The figure shows three views and two pictorial views of one solid part (mm, origin at its lowest corner). Answer the questions. Give positions to 0.01 mm unless a question says otherwise; leave off trailing zeros. Loops run counter-clockwise (first coordinate to the right, second up) from the corner with the lowest first, then second, coordinate; pieces in that order, holes last. Notation, with made-up numbers: M 30,19 L 55,19 A18 ccw 55,38 Z; hole C -23,-21 d6. An arc over 180 degrees is marked long. Write item = value, one per line. Start each with the question number.
1. Section B-B on x = 62.5 is taken. Determine the outline of the cut face in (y, z) (1 decimal).
2. Consider L1, parallel to X at y = 4, z = 78.5 (1 decimal); L2, parallel to X at y = 1.25, z = 56.5 (1 decimal); L3, parallel to Z at x = 62.5, y = 0.8 (1 decimal). Determine where each line is inside the solid, lowest interval first. Write a range as [from, to].
3. Section A-A on z = 44.25 is taken. Determine the outline of the cut face in (x, y).
4. Section C-C on z = 61 is taken. Determine the outline of the cut face in (x, y).
5. The mould has two halves that part along X. Classify the marked faces 1, 2, 3 and 4: released by +X, released by -X, zero draft, split by the parting line, or undercut.
6. Flat-ended cylindrical pins translate along their axes: pin 1 Ø5 at (x, z) = (16, 67) entering from +Y; pin 2 Ø1.8 at (x, z) = (63.5, 76.5) entering from +Y; pin 3 Ø9.5 at (x, z) = (37.91, 80.2) entering from -Y; pin 4 Ø4 at (x, y) = (25, 2.5) entering from -Z. Find the tip coordinate at first contact, or state that the pin passes through.
7. Section D-D on y = 3.75 is taken. Give the number of separate pieces and of enclosed holes in the cut face, plus the area to 3 significant figures.
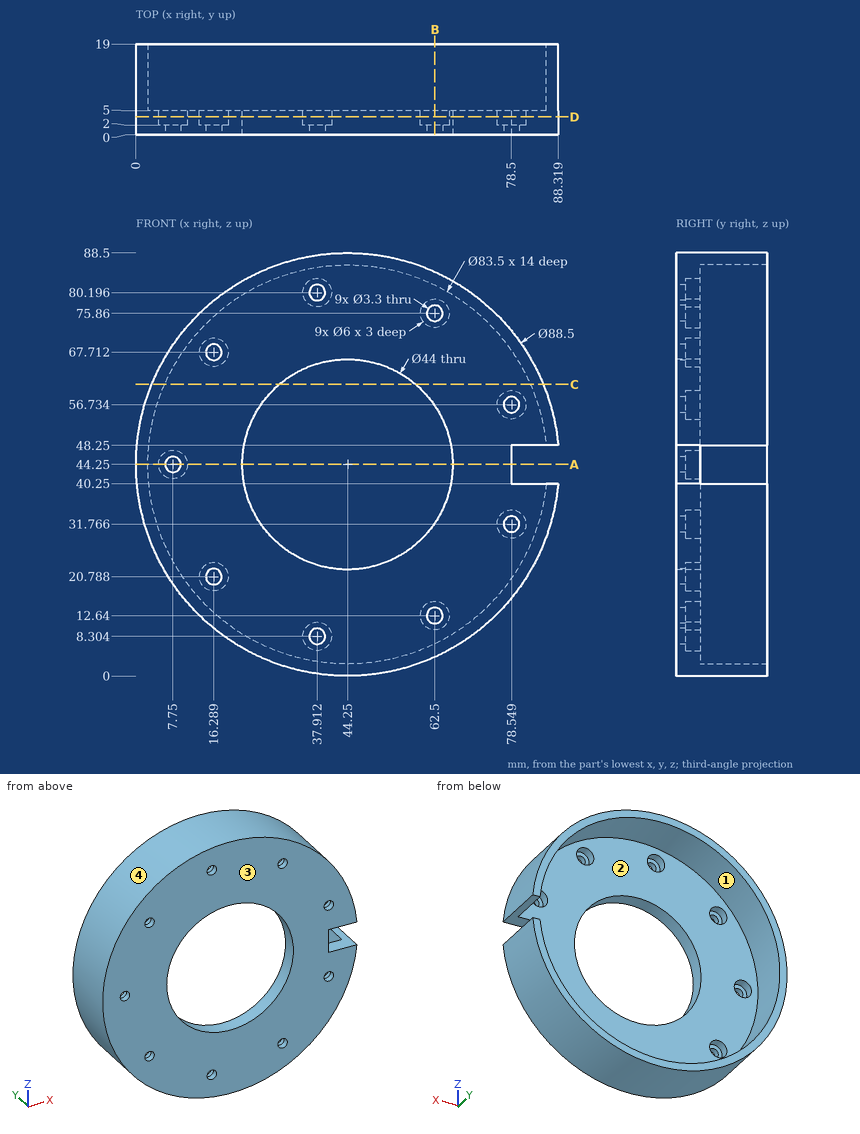
Verdict:
q1.outline = M 0,3.9 L 19,3.9 L 19,6.7 L 5,6.7 L 5,9.6 L 2,9.6 L 2,11 L 0,11 Z; M 0,14.3 L 2,14.3 L 2,15.6 L 5,15.6 L 5,32 L 0,32 Z; M 0,56.5 L 5,56.5 L 5,72.9 L 2,72.9 L 2,74.2 L 0,74.2 Z; M 0,77.5 L 2,77.5 L 2,78.9 L 5,78.9 L 5,81.8 L 19,81.8 L 19,84.6 L 0,84.6 Z
q2.L1 = [16.2, 35.4], [40.4, 61.1], [63.9, 72.3]
q2.L2 = [1.7, 26], [62.5, 76.9], [80.2, 86.8]
q2.L3 = [3.9, 11], [14.3, 32], [56.5, 74.2], [77.5, 84.6]
q3.outline = M 0,0 L 6.1,0 L 6.1,2 L 4.75,2 L 4.75,5 L 2.5,5 L 2.5,19 L 0,19 Z; M 9.4,0 L 22.25,0 L 22.25,5 L 10.75,5 L 10.75,2 L 9.4,2 Z; M 66.25,0 L 78.5,0 L 78.5,5 L 66.25,5 Z
q4.outline = M 3.29,0 L 29.99,0 L 29.99,5 L 6.01,5 L 6.01,19 L 3.29,19 Z; M 58.51,0 L 85.21,0 L 85.21,19 L 82.49,19 L 82.49,5 L 58.51,5 Z
q5.face_1 = undercut
q5.face_2 = undercut
q5.face_3 = zero draft
q5.face_4 = split by the parting line
q6.pin_1 = 5
q6.pin_2 = 2
q6.pin_3 = 0
q6.pin_4 = 3.5
q7.separate_pieces = 1
q7.enclosed_holes = 10
q7.area = 4,300 mm2
